Geometry check sheet. Reference: the model listing, model coordinates, mm. A direction names the side the tool comes from. Coordinates: 2 decimals unless noted, no trailing zeros. Loops run counter-clockwise (first coordinate to the right, second up) from the corner with the lowest first, then second, coordinate; pieces in that order, holes last.
from build123d import *

# Parameters (mm, degrees)
SKETCH_W        = 54
SKETCH_H        = 82
PAD_DEPTH       = 25
SKETCH001_W     = 50
SKETCH001_H     = 78
POCKET_DEPTH    = 22
SKETCH002_R     = 2.75
PAD001_DEPTH    = 4
SKETCH003_R     = 1.75
POCKET001_DEPTH = 23
CHAMFER_SIZE    = 1.5
FILLET_R        = 1


with BuildPart() as part:
    # Sketch → Pad (new body)
    with BuildSketch(Plane.XY):
        Rectangle(SKETCH_W, SKETCH_H)
    extrude(amount=PAD_DEPTH)

    # Sketch001 (on Face6 of Pad) → Pocket (cut)
    with BuildSketch(Plane.XY.offset(25)):
        Rectangle(SKETCH001_W, SKETCH001_H)
    extrude(amount=-POCKET_DEPTH, mode=Mode.SUBTRACT)

    # Sketch002 (on Face11 of Pocket) → Pad001 (join)
    with BuildSketch(Plane.XY.offset(3)):
        with Locations((-20.32, 34.29)):
            Circle(SKETCH002_R)
        with Locations((20.32, 34.29)):
            Circle(SKETCH002_R)
        with Locations((-20.32, -34.29)):
            Circle(SKETCH002_R)
        with Locations((20.32, -34.29)):
            Circle(SKETCH002_R)
    extrude(amount=PAD001_DEPTH)

    # Sketch003 (on Face4 of Pad001) → Pocket001 (cut)
    with BuildSketch(Plane(origin=(0, 0, 0), x_dir=(1, 0, 0), z_dir=(0, 0, -1))):
        with Locations((20.32, -34.29)):
            Circle(SKETCH003_R)
        with Locations((-20.32, -34.29)):
            Circle(SKETCH003_R)
        with Locations((-20.32, 34.29)):
            Circle(SKETCH003_R)
        with Locations((20.32, 34.29)):
            Circle(SKETCH003_R)
    extrude(amount=-POCKET001_DEPTH, mode=Mode.SUBTRACT)

    # Chamfer
    chamfer_edges = [part.edges().sort_by_distance(p)[0] for p in [
        (18.57, 34.29, 0),
        (-22.07, 34.29, 0),
        (-22.07, -34.29, 0),
        (18.57, -34.29, 0),
    ]]
    chamfer(chamfer_edges, length=CHAMFER_SIZE)

    # Fillet
    fillet_edges = [part.edges().sort_by_distance(p)[0] for p in [
        (0, 41, 0),
        (27, 41, 12.5),
        (27, 0, 0),
        (0, -41, 0),
        (-27, 0, 0),
        (-27, 41, 12.5),
        (27, -41, 12.5),
        (-27, -41, 12.5),
    ]]
    fillet(fillet_edges, radius=FILLET_R)


solid = part.part
1) Depth check by flat-ended pin: pin 1 (1.6 mm diameter, centred on x = 21, y = 35, fed in from +Z); pin 2 (1.6 mm diameter, centred on x = -19.5, y = -34, fed in from +Z); pin 3 (4 mm diameter, centred on x = 20.32, y = -34.29, fed in from -Z); pin 4 (4 mm diameter, centred on x = 17.5, y = 14, fed in from +Z). Enter the tip coordinate at first touch or a pass-through.
Data:
pin 1: stops at z = 7
pin 2: passes through
pin 3: stops at z = 1.25
pin 4: stops at z = 3
2) Access from +Z, -Z, +X, -X, +Y, -Y to the whole of each face (thin tool, end or side, straight path). Record for faces 5 (the cylindrical face through (-19.51, 35.84, 4.21)), 6 (the flat face through (25, -1, 14)).
Data:
face 5: +Z, -Z
face 6: +Z
3) Section check A-A on z = 4.75. Count the separate pieces of the cut face and the enclosed holes in it, and give its area (3 significant figures).
Data:
separate pieces: 5
enclosed holes: 5
area: 584 mm2
4) Section check D-D on z = 22.25. Record the cut outline in (x, y), and give its area (3 significant figures).
Data:
outline: (-27, -40) arc R1 ccw to (-26, -41) - (26, -41) arc R1 ccw to (27, -40) - (27, 40) arc R1 ccw to (26, 41) - (-26, 41) arc R1 ccw to (-27, 40) - close; hole (-25, -39) - (25, -39) - (25, 39) - (-25, 39) - close
area: 527 mm2
5) Mould release check, pull along Y, two halves, no side actions. Record for faces 1 (the flat face through (-25, -1, 14)), 2 (the flat face through (0, -39, 14)), 3 (the flat face through (0, -41, 13)), 4 (the flat face through (27, -1, 13)): +Y half, -Y half, draft (parallel to the pull), parting line (faces both ways), or undercut.
Data:
face 1: undercut
face 2: undercut
face 3: -Y half
face 4: draft
6) Material ranges on probe 1 along Y at (x, z) = (-20.32, 5.45); probe 2 along Y at (x, z) = (-20.32, 2.9); probe 3 along X at (y, z) = (-34.29, 2.8), recorded low to high.
Data:
probe 1: y = -41 to -39, -37.04 to -36.04, -32.54 to -31.54, 31.54 to 32.54, 36.04 to 37.04, 39 to 41
probe 2: y = -41 to -36.04, -32.54 to 32.54, 36.04 to 41
probe 3: x = -27 to -22.07, -18.57 to 18.57, 22.07 to 27
